Verification items for the finished model (mm, model axes). Face numbers are marked on the shaded views. A direction names the side the tool comes from. Give positions to 0.01 mm unless a question says otherwise; leave off trailing zeros. Order: outer loops, then holes, each group sorted by start corner. A loop starts at its lowest first (then second) coordinate and runs counter-clockwise, first axis right, second up. Notation, with made-up numbers: (18, 10) -> (24, 10) arc R30 ccw to (24, 36) -> close; hole circle Ø7 at (5.5, 0). An arc over 180 degrees is marked (long way). Return JSON: item names as keys, results as strings. Group by question number.
(1) Cross-section at D-D on y = -2.5. Enter the section's corners in (x, z), then the cut area to 3 significant figures.
(2) Cross-section at A-A on y = 3.75. Enter the section's corners in (x, z), then the cut area to 3 significant figures.
(3) Release check for a two-part mould opening along Y. For the marked faces 6, 7, 8 and 9 record: pulls with the +Y half, pulls with the -Y half, needs draft (parallel to the pull), parting line crosses it, or undercut.
(4) Cross-section at B-B on x = 0. Enter the section's corners in (y, z), then the cut area to 3 significant figures.
(5) Thickness scan on line 1 along Y through (x, z) = (3, -3.5); line 2 along X through (y, z) = (4.75, -0.5); line 3 along Y through (x, z) = (1.5, 4). Record the ranges inside material, lowest first.
(6) Cross-section at C-C on z = 0.25. Enter the section's corners in (x, y).
(7) Tool access check on the marked faces 1, 2, 3, 4 and 5. Record the directions out of +Z, -Z, +X, -X, +Y, -Y that give a thin tool (end or side, any length) a straight path to the whole face; none if there is none.
(8) Depth check by flat-ended pin: pin 1 Ø0.6 at (x, y) = (0.5, -1.5) entering from -Z; pin 2 Ø0.9 at (x, y) = (5.5, -1.5) entering from +Z; pin 3 Ø0.9 at (y, z) = (7, 0) entering from -X. Enter the tip coordinate at first touch or a pass-through.
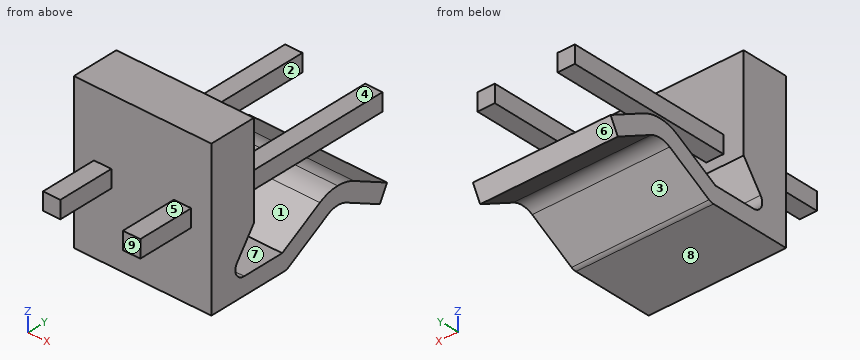
from build123d import *

# Parameters (mm, degrees)
CROQUIS1_W                   = 8.74
CROQUIS1_H                   = 9.7
CROQUIS1_W_2                 = 1.1
CROQUIS1_H_2                 = 1.1
SALIENTE_EXTRUIR1_DEPTH      = 3
CROQUIS2_W                   = 8.74
CROQUIS2_H                   = 3
SALIENTE_EXTRUIR2_DEPTH      = 9.4
CORTAR_EXTRUIR1_START        = -8.74
CORTAR_EXTRUIR1_DEPTH        = 8.74
SALIENTE_EXTRUIR3_DEPTH      = 13.5
SALIENTE_EXTRUIR3_DEPTH_BACK = 3.6
CROQUIS5_W                   = 1.1
CROQUIS5_H                   = 1.1


# Read off the part's stored shape, not the designer's step: Cortar-Extruir1
with BuildPart() as part:
    # Croquis1 → Saliente-Extruir1 (new body)
    with BuildSketch(Plane(origin=(0, 0, 0), x_dir=(1, 0, 0), z_dir=(0, 1, 0))):
        with Locations((2.54, 0.1)):
            Rectangle(CROQUIS1_W, CROQUIS1_H)
        Rectangle(CROQUIS1_W_2, CROQUIS1_H_2, mode=Mode.SUBTRACT)
        with Locations((5.08, 0)):
            Rectangle(CROQUIS1_W_2, CROQUIS1_H_2, mode=Mode.SUBTRACT)
    extrude(amount=SALIENTE_EXTRUIR1_DEPTH)

    # Croquis2 → Saliente-Extruir2 (add)
    with BuildSketch(Plane(origin=(0, 3, 0), x_dir=(1, 0, 0), z_dir=(0, 1, 0))):
        with Locations((2.54, 3.45)):
            Rectangle(CROQUIS2_W, CROQUIS2_H)
    extrude(amount=SALIENTE_EXTRUIR2_DEPTH)

    # Cortar-Extruir1 outline → Cortar-Extruir1 (cut)
    with BuildSketch(Plane.ZY.offset(1.83).offset(CORTAR_EXTRUIR1_START)):
        with BuildLine():
            Line((-1.95, 3), (-1.95, 8.9155089))
            ThreePointArc((-1.95, 8.9155089), (-2.036358841, 8.267369623), (-2.28940975, 7.664453701))
            Line((-2.28940975, 7.664453701), (-3.85, 5))
            Line((-3.85, 5), (-3.85, 2.319959731))
            ThreePointArc((-3.85, 2.319959731), (-3.508458272, 1.760049187), (-2.854318236, 1.807497933))
            Line((-2.854318236, 1.807497933), (-1.184444515, 3))
            Line((-1.184444515, 3), (-1.95, 3))
        make_face()
        with BuildLine():
            Line((-1.95, 12.4), (-3.455311447, 12.4))
            Line((-3.455311447, 12.4), (-2.232277415, 10.063467416))
            ThreePointArc((-2.232277415, 10.063467416), (-2.021605007, 9.506586157), (-1.95, 8.9155089))
            Line((-1.95, 8.9155089), (-1.95, 12.4))
        make_face()
        with BuildLine():
            Line((-3.206840185, 9.553342522), (-4.429874218, 11.889875107))
            Line((-4.429874218, 11.889875107), (-3.455311447, 12.4))
            Line((-3.455311447, 12.4), (-4.95, 12.4))
            Line((-4.95, 12.4), (-4.95, 5.130923429))
            ThreePointArc((-4.95, 5.130923429), (-4.928460036, 5.292584893), (-4.865343077, 5.442966568))
            Line((-4.865343077, 5.442966568), (-3.238584298, 8.220392257))
            ThreePointArc((-3.238584298, 8.220392257), (-3.050389859, 8.882763545), (-3.206840185, 9.553342522))
        make_face()
    extrude(amount=CORTAR_EXTRUIR1_DEPTH, mode=Mode.SUBTRACT)

    # Croquis5 → Saliente-Extruir3 (add, two sides: drawn at the far end of the back side and taken through both)
    with BuildSketch(Plane(origin=(0, 0, 0), x_dir=(1, 0, 0), z_dir=(0, 1, 0)).offset(-SALIENTE_EXTRUIR3_DEPTH_BACK)):
        with Locations((5.08, 0)):
            Rectangle(CROQUIS5_W, CROQUIS5_H)
        Rectangle(CROQUIS5_W, CROQUIS5_H)
    extrude(amount=SALIENTE_EXTRUIR3_DEPTH + SALIENTE_EXTRUIR3_DEPTH_BACK)


solid = part.part
Verdict:
{
 "1": {"outline": "(-0.55, -0.55) -> (0.55, -0.55) -> (0.55, 0.55) -> (-0.55, 0.55) -> close; (4.53, -0.55) -> (5.63, -0.55) -> (5.63, 0.55) -> (4.53, 0.55) -> close", "area": "2.42 mm²"},
 "2": {"outline": "(-1.83, -4.95) -> (6.91, -4.95) -> (6.91, -3.85) -> (-1.83, -3.85) -> close; (-0.55, -0.55) -> (0.55, -0.55) -> (0.55, 0.55) -> (-0.55, 0.55) -> close; (4.53, -0.55) -> (5.63, -0.55) -> (5.63, 0.55) -> (4.53, 0.55) -> close", "area": "12.0 mm²"},
 "3": {"face 6": "pulls with the +Y half", "face 7": "undercut", "face 8": "needs draft", "face 9": "pulls with the -Y half"},
 "4": {"outline": "(-3.6, -0.55) -> (0, -0.55) -> (0, -4.95) -> (5.13, -4.95) arc R0.62 ccw to (5.44, -4.87) -> (8.22, -3.24) arc R1.38 cw to (9.55, -3.21) -> (11.89, -4.43) -> (12.4, -3.46) -> (10.06, -2.23) arc R2.48 ccw to (7.66, -2.29) -> (5, -3.85) -> (2.32, -3.85) arc R0.63 cw to (1.81, -2.85) -> (3, -1.18) -> (3, -0.55) -> (13.5, -0.55) -> (13.5, 0.55) -> (3, 0.55) -> (3, 4.75) -> (0, 4.75) -> (0, 0.55) -> (-3.6, 0.55) -> close", "area": "53.4 mm²"},
 "5": {"line 1": "0 to 1.76, 5.6 to 7.77, 10.11 to 12.38", "line 2": "-0.55 to 0.55, 4.53 to 5.63", "line 3": "0 to 3"},
 "6": {"outline": "(-1.83, 0) -> (-0.55, 0) -> (-0.55, -3.6) -> (0.55, -3.6) -> (0.55, 0) -> (4.53, 0) -> (4.53, -3.6) -> (5.63, -3.6) -> (5.63, 0) -> (6.91, 0) -> (6.91, 3) -> (5.63, 3) -> (5.63, 13.5) -> (4.53, 13.5) -> (4.53, 3) -> (0.55, 3) -> (0.55, 13.5) -> (-0.55, 13.5) -> (-0.55, 3) -> (-1.83, 3) -> close"},
 "7": {"face 1": "+X, -X", "face 2": "+Z, +Y", "face 3": "-Z, +X, -X", "face 4": "+Z, +X, -X, +Y", "face 5": "+Z, +X, -X, -Y"},
 "8": {"pin 1": "z = -0.55", "pin 2": "z = 0.55", "pin 3": "x = -0.55"}
}
